Here's how the part is built. I have some questions about the finished solid (model axes, mm). Face numbers are marked on the shaded views. Round coordinates to 2 decimals unless told otherwise and drop trailing zeros. Write each loop counter-clockwise with the first axis right and the second up, starting at its lowest first coordinate (ties: lowest second). Pieces come first, ordered by that corner, then holes. Notation, with made-up numbers: (6.5, -11) -> (56.5, -11) arc R21 cw to (56.5, 1) -> close; hole circle Ø3 at (81.25, 24.25). An arc over 180 degrees is marked (long way). Answer as CSV lines item,"result".
```python
from build123d import *

# Parameters (mm, degrees)
SKETCH1_W           = 10
SKETCH1_H           = 10
BOSS_EXTRUDE1_DEPTH = 7
SKETCH2_R           = 1.5
CUT_EXTRUDE1_DEPTH  = 3
SKETCH3_R           = 1.25
SKETCH3_R_2         = 1
BOSS_EXTRUDE2_DEPTH = 2
FILLET1_R           = 0.2


with BuildPart() as part:
    # Sketch1 → Boss-Extrude1 (new body)
    with BuildSketch(Plane.XY):
        Rectangle(SKETCH1_W, SKETCH1_H)
    extrude(amount=BOSS_EXTRUDE1_DEPTH)

    # Sketch2 → Cut-Extrude1 (cut)
    with BuildSketch(Plane.XY.offset(7)):
        Circle(SKETCH2_R)
    extrude(amount=-CUT_EXTRUDE1_DEPTH, mode=Mode.SUBTRACT)

    # Sketch3 → Boss-Extrude2 (add)
    with BuildSketch(Plane.XY.offset(4)):
        Circle(SKETCH3_R)
        Circle(SKETCH3_R_2, mode=Mode.SUBTRACT)
    extrude(amount=BOSS_EXTRUDE2_DEPTH)

    # Fillet1
    fillet1_edges = [part.edges().sort_by_distance(p)[0] for p in [
        (-5, 5, 3.5),
        (5, 5, 3.5),
        (5, -5, 3.5),
        (-5, -5, 3.5),
    ]]
    fillet(fillet1_edges, radius=FILLET1_R)


solid = part.part
```
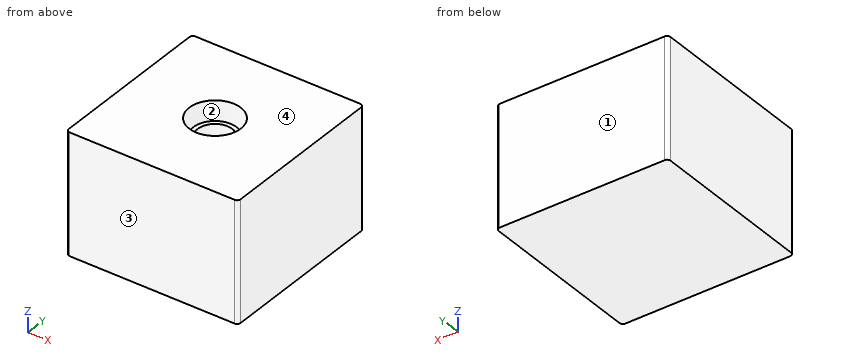
1. Suppose I cut it at A-A on z = 4.25. Please give me the cut outline in (x, y).
Numbers:
outline,"(-5, -4.8) arc R0.2 ccw to (-4.8, -5) -> (4.8, -5) arc R0.2 ccw to (5, -4.8) -> (5, 4.8) arc R0.2 ccw to (4.8, 5) -> (-4.8, 5) arc R0.2 ccw to (-5, 4.8) -> close; circle Ø2.5 at (0, 0); hole circle Ø3 at (0, 0); hole circle Ø2 at (0, 0)"
2. Suppose I cut it at B-B on y = 0. Please give me the cut outline in (x, z).
Numbers:
outline,"(-5, 0) -> (5, 0) -> (5, 7) -> (1.5, 7) -> (1.5, 4) -> (1.25, 4) -> (1.25, 6) -> (1, 6) -> (1, 4) -> (-1, 4) -> (-1, 6) -> (-1.25, 6) -> (-1.25, 4) -> (-1.5, 4) -> (-1.5, 7) -> (-5, 7) -> close"
3. Suppose I cut it at D-D on z = 6.25. Please give me the cut outline in (x, y), and give its area (3 significant figures).
Numbers:
outline,"(-5, -4.8) arc R0.2 ccw to (-4.8, -5) -> (4.8, -5) arc R0.2 ccw to (5, -4.8) -> (5, 4.8) arc R0.2 ccw to (4.8, 5) -> (-4.8, 5) arc R0.2 ccw to (-5, 4.8) -> close; hole circle Ø3 at (0, 0)"
area,"92.9 mm^2"
4. For pin 1 Ø0.9 at (x, y) = (0, 0) entering from +Z; pin 2 Ø1.2 at (x, y) = (-0.5, -0.5) entering from +Z; pin 3 Ø5 at (x, y) = (-1, 1) entering from +Z, each with a flat end and sliding along its axis, tell me the tip position at first contact or that it passes through.
Numbers:
pin 1,"stops at z = 4"
pin 2,"stops at z = 6"
pin 3,"stops at z = 7"
5. If we mould it in two halves opening along Y, with no side actions, what happens to the marked faces 1, 2, 3 and 4? For each: released by +Y, released by -Y, zero draft, split by the parting line, or undercut.
Numbers:
face 1,"released by +Y"
face 2,"undercut"
face 3,"released by -Y"
face 4,"zero draft"
6. If I drill on line 1 (Y direction, x = 0, z = 5.65); line 2 (Y direction, x = 0, z = 6.15), over which ranges is the centre line in solid material (lowest first)?
Numbers:
line 1,"y = -5 to -1.5, -1.25 to -1, 1 to 1.25, 1.5 to 5"
line 2,"y = -5 to -1.5, 1.5 to 5"
